Autodesk Inventor part; units mm, degrees
ref_plane "YZ Plane" through (0, 0, 0) normal (1, 0, 0) x (0, 1, 0)
ref_plane "XZ Plane" through (0, 0, 0) normal (0, 1, 0) x (-1, 0, 0)
ref_plane "XY Plane" through (0, 0, 0) normal (0, 0, 1) x (1, 0, 0)
sketch "Esquisse1" plane through (0, 0, 0) normal (0, 0, 1) x (1, 0, 0)
  line L0 (20, 0) -> (-20, 0) construction
  line L1 (20, -6.1) -> (-20, -6.1)
  line L2 (-20, 6.1) -> (20, 6.1)
  arc A0 (20, -6.1) -> (20, 6.1) centre (20, 0) ccw
  arc A1 (-20, 6.1) -> (-20, -6.1) centre (-20, 0) ccw
  circle A2 centre (-20, 0) radius 1.55
  circle A3 centre (20, 0) radius 2.1
  line L3 (-5, -6.1) -> (5, -6.1)
  line L4 (5, -6.1) -> (5, 6.1)
  line L5 (5, 6.1) -> (-5, 6.1)
  line L6 (-5, 6.1) -> (-5, -6.1)
  line L7 (-5, -6.1) -> (5, 6.1) construction
  line L8 (5, -6.1) -> (-5, 6.1) construction
  point P0 (0, 0)
  dimension "d0" = 40
  dimension "d1" = 3.1
  dimension "d5" = 4.2
  dimension "d6" = 4
  dimension "d12" = 10
extrude "Extrusion1" add sketch "Esquisse1" along normal blind 5.5 contours L1 L6 L2 L4 | L1 A1 L2 L6
extrude "Extrusion4" add sketch "Esquisse1" against normal blind 5 contours L1 L4 L2 A0 | L1 L6 L2 L4
fillet "Congé1" radius 1.5 4 edges at (-5, 6.1, -2.5) (-5, -6.1, -2.5) (5, -6.1, 2.75) (5, 6.1, 2.75)
properties part number "Biellette support-doigts"
Input: part model. Units: mm. Frame: model coordinates. A direction names the side the tool comes from. Coordinates: 2 decimals unless noted, no trailing zeros. Loops run counter-clockwise (first coordinate to the right, second up) from the corner with the lowest first, then second, coordinate; pieces in that order, holes last. Notation, with made-up numbers: (-37.5, 14.25) - (-27.5, 14.25) arc R14 cw to (-27.5, 26.25) - close; hole circle Ø11 at (-34.5, 28.5). An arc over 180 degrees is marked (long way). Answer in a Markdown table with one row per item.
(1) Cut plane C-C on x = 21. Output: boundary loops of the cut face in (y, z), plus the area to 3 significant figures.
Model answer:
| item | result |
|---|---|
| outline | (-6.02, -5) - (-1.85, -5) - (-1.85, 0) - (-6.02, 0) - close; (1.85, -5) - (6.02, -5) - (6.02, 0) - (1.85, 0) - close |
| area | 41.7 mm² |
(2) Cut plane A-A on y = 0. Output: boundary loops of the cut face in (x, z), plus the area to 4 significant figures.
Model answer:
| item | result |
|---|---|
| outline | (-26.1, 0) - (-21.55, 0) - (-21.55, 5.5) - (-26.1, 5.5) - close; (-18.45, 0) - (-5, 0) - (-5, -5) - (17.9, -5) - (17.9, 0) - (5, 0) - (5, 5.5) - (-18.45, 5.5) - close; (22.1, -5) - (26.1, -5) - (26.1, 0) - (22.1, 0) - close |
| area | 288.5 mm² |
(3) Cut plane B-B on z = 3.5. Output: boundary loops of the cut face in (x, y), plus the area to 3 significant figures.
Model answer:
| item | result |
|---|---|
| outline | (-20, -6.1) - (3.5, -6.1) arc R1.5 ccw to (5, -4.6) - (5, 4.6) arc R1.5 ccw to (3.5, 6.1) - (-20, 6.1) arc R6.1 ccw to start; hole circle Ø3.1 at (-20, 0) |
| area | 355 mm² |
(4) Material intervals for L1, parallel to Y at x = 20, z = -2.95; L2, parallel to Y at x = -20, z = 1.1; L3, parallel to Z at x = 17.5, y = 4, sorted ascending. Write a range as from..to.
Model answer:
| item | result |
|---|---|
| L1 | y = -6.1..-2.1, 2.1..6.1 |
| L2 | y = -6.1..-1.55, 1.55..6.1 |
| L3 | z = -5..0 |
(5) Pin query (flat end, axial travel): P1, Ø6, axis at x = -15.5, y = 0.5, coming from the -Z side; P2, Ø3, axis at y = -0.5, z = -0.5, coming from the +X side; P3, Ø1.5, axis at x = 6.5, y = 4.5, coming from the +Z side; P4, Ø6, axis at y = 4, z = -1.5, coming from the -X side. Return the tip coordinate at first contact, or that it passes through.
Model answer:
| item | result |
|---|---|
| P1 | stops at z = 0 |
| P2 | stops at x = 26.1 |
| P3 | stops at z = 0 |
| P4 | stops at x = -25.94 |
(6) Cut plane D-D on z = -4. Output: boundary loops of the cut face in (x, y), plus the area to 3 significant figures.
Model answer:
| item | result |
|---|---|
| outline | (-5, -4.6) arc R1.5 ccw to (-3.5, -6.1) - (20, -6.1) arc R6.1 ccw to (20, 6.1) - (-3.5, 6.1) arc R1.5 ccw to (-5, 4.6) - close; hole circle Ø4.2 at (20, 0) |
| area | 349 mm² |
(7) Set-up query: faces 5 (the face through (4.57, 5.65, 2.79)), 6 (the face through (5, 0, 3)), 7 (the face through (-4.57, 5.65, -2.54)), 8 (the face through (-4.55, -5.67, -2.54)), 9 (the face through (4.55, -5.67, 2.79)). Return all of +Z, -Z, +X, -X, +Y, -Y with unobstructed straight access to the full face (end or side cutting, diameter ignored); none if empty.
Model answer:
| item | result |
|---|---|
| face 5 | +Z, +X, +Y |
| face 6 | +Z, +X, +Y, -Y |
| face 7 | -Z, -X, +Y |
| face 8 | -Z, -X, -Y |
| face 9 | +Z, +X, -Y |
(8) Mould query, pull axis X, two halves, no side actions, for faces 1 (the face through (26.1, -0.1, -2.5)), 2 (the face through (0, 6.1, 0)), 3 (the face through (-5, 0, -2)), 4 (the face through (22.003, 0.631, -2.465)). Classes: pulls with the +X half, pulls with the -X half, needs draft (parallel to the pull), parting line crosses it, or undercut.
Model answer:
| item | result |
|---|---|
| face 1 | pulls with the +X half |
| face 2 | needs draft |
| face 3 | pulls with the -X half |
| face 4 | undercut |
